For this review, take the finished solid that the model builds, in its own axes (mm). A direction names the side the tool comes from. Give positions to 0.01 mm unless a question says otherwise; leave off trailing zeros. Loops run counter-clockwise (first coordinate to the right, second up) from the corner with the lowest first, then second, coordinate; pieces in that order, holes last. Notation, with made-up numbers: (56, 17.25) - (65, 17.25) arc R12 cw to (65, 26.25) - close; hole circle Ø8 at (62, 79). An arc over 180 degrees is marked (long way). Use CSV: the item, a comma, the result in double quotes. Start each with the question number.
1. Wall thickness on line 1 (X direction, y = 0.5, z = -18); line 2 (X direction, y = -1, z = -23.5); line 3 (X direction, y = 3, z = -22.5): over which ranges is each line inside the solid? List them lowest first.
2. For faces 1 (the cylindrical face through (0.37, -0.06, -45.34)), 2 (the cylindrical face through (12.476, -0.632, 52.395)), list the 3-axis set-ups (+Z, -Z, +X, -X, +Y, -Y) from which the entire face can be reached by the end or side of a thin tool; tool diameter is ignored.
3. Take a section at B-B on z = 2.5. Give the boundary of the cut face in (x, y).
4. Take a section at C-C on x = -10.5. Give the boundary of the cut face in (y, z), plus the area to 3 significant figures.
5. Mouldability with a two-part tool opening along Y and no side actions: class faces 3 (the cylindrical face through (0.37, -0.06, 48.66)), 4 (the flat face through (32, -4, 25)), 5 (the cylindrical face through (-15.524, -0.632, 52.395)) as pulls with the +Y half, pulls with the -Y half, needs draft (parallel to the pull), parting line crosses it, or undercut.
6. Take a section at A-A on z = 23.5. Give the boundary of the cut face in (x, y), plus the area to 3 significant figures.
7. Take a section at D-D on x = 47. Give the boundary of the cut face in (y, z).
8. For pin 1 (4 mm diameter, centred on x = 0, z = -47, fed in from +Y); pin 2 (2 mm diameter, centred on x = -14, y = 0, fed in from +Z); pin 3 (3 mm diameter, centred on y = 0, z = -36.5, fed in from +X); pin 4 (1.5 mm diameter, centred on x = -40, y = 1, fed in from +Z), all flat-tipped, find the tip position at first contact; note any pin that passes through.
```python
from build123d import *

# Parameters (mm, degrees)
SKETCH_2_R                  = 40
EXTRUDE_1_DEPTH             = 4
HOLE_WIZARD_M3_1_D          = 3.4
HOLE_WIZARD_M4_1_AT_2_COUNT = 2
HOLE_WIZARD_M4_1_AT_2_PITCH = 28
HOLE_WIZARD_M4_3_D          = 3.3
HOLE_WIZARD_M4_3_DEPTH      = 15
HOLE_WIZARD_M4_3_TIP        = 0.991420021
HOLE_WIZARD_M4_2_D          = 4.3


with BuildPart() as part:
    # 草图2 → 凸台-拉伸1 (new, symmetric)
    with BuildSketch(Plane(origin=(0, 0, 0), x_dir=(1, 0, 0), z_dir=(0, 1, 0))):
        Polygon((23, 61.852813742), (-23, 61.852813742), (-74.618795027, 10.234018716), (-35, -60), (35, -60), (74.618795027, 10.234018716), align=None)
        with Locations(Location((0, 0, 0), (0, 0, 270))):
            Circle(SKETCH_2_R, mode=Mode.SUBTRACT)
    extrude(amount=EXTRUDE_1_DEPTH, both=True)

    # M3 间隙孔1 (through all)
    with Locations(Plane(origin=(0, 4, 0), x_dir=(1, 0, 0), z_dir=(0, 1, 0))):
        with Locations((0, 47), (40.703193978, 23.5), (40.703193978, -23.5), (0, -47), (-40.703193978, -23.5), (-40.703193978, 23.5)):
            Hole(HOLE_WIZARD_M3_1_D / 2)

    # 草图7 → Hole Wizard M4 _1 (revolve, cut)
    with BuildSketch(Plane(origin=(38.820162287, 0, -46.032651455), x_dir=(-0.7071067811865476, 0, -0.7071067811865476), z_dir=(0, 1, 0))):
        Polygon((0, 0), (0, 12.991420021), (1.65, 12), (1.65, 0), align=None)
    hole_wizard_m4_1 = revolve(axis=Axis((43.310290348, 0, -50.522779516), (-0.7071067811865476, 0, 0.7071067811865476)), mode=Mode.SUBTRACT)

    # Hole Wizard M4 _1 at 2: Hole Wizard M4 _1 ×2
    with Locations(*[Vector(0.7071067811865476, 0, 0.7071067811865476) * (i * HOLE_WIZARD_M4_1_AT_2_PITCH) for i in range(1, HOLE_WIZARD_M4_1_AT_2_COUNT)]):
        add(hole_wizard_m4_1, mode=Mode.SUBTRACT)

    # 镜向1: Hole Wizard M4 _1 across plane
    add(hole_wizard_m4_1.mirror(Plane(origin=(0, 0, 0), x_dir=(0, 0, 1), z_dir=(1, 0, 0))), mode=Mode.SUBTRACT)

    # 镜向1 copy 1 sketch → 镜向1 copy 1 (revolve, cut)
    with BuildSketch(Plane(origin=(-58.61915216, 0, -26.233661582), x_dir=(0.7071067811865476, 0, -0.7071067811865476), z_dir=(0, 1, 0))):
        Polygon((0, 0), (0, -12.991420021), (1.65, -12), (1.65, 0), align=None)
    revolve(axis=Axis((-63.109280221, 0, -30.723789643), (-0.7071067811865476, 0, -0.7071067811865476)), mode=Mode.SUBTRACT)

    # M4 螺纹孔3
    with Locations(Plane.XY.offset(60)):
        with Locations((14, 0), (-14, 0)):
            Hole(HOLE_WIZARD_M4_3_D / 2, depth=HOLE_WIZARD_M4_3_DEPTH)
            with Locations((0, 0, -(HOLE_WIZARD_M4_3_DEPTH + HOLE_WIZARD_M4_3_TIP / 2))):  # 118° drill point
                Cone(0, HOLE_WIZARD_M4_3_D / 2, HOLE_WIZARD_M4_3_TIP, mode=Mode.SUBTRACT)

    # M4 间隙孔2 (through all)
    with Locations(Plane(origin=(0, 4, 0), x_dir=(1, 0, 0), z_dir=(0, 1, 0))):
        with Locations((0, 56), (0, -56)):
            Hole(HOLE_WIZARD_M4_2_D / 2)


solid = part.part
```
Check result:
1,line 1,"x = -66.85 to -52.61, -49.27 to -35.72, 35.72 to 49.27, 52.61 to 66.85"
1,line 2,"x = -61.35 to -57.74, -54.03 to -42.4, -39 to -32.37, 32.37 to 39, 42.4 to 54.03, 57.74 to 61.35"
1,line 3,"x = -62.35 to -42.08, -39.33 to -33.07, 33.07 to 39.33, 42.08 to 62.35"
2,face 1,"+Y, -Y"
2,face 2,"+Z"
3,outline,"(-67.44, -4) - (-39.92, -4) - (-39.92, 4) - (-67.44, 4) - close; (39.92, -4) - (67.44, -4) - (67.44, 4) - (39.92, 4) - close"
4,outline,"(-4, -61.85) - (4, -61.85) - (4, -38.6) - (-4, -38.6) - close; (-4, 38.6) - (4, 38.6) - (4, 60) - (-4, 60) - close"
4,area,"357 mm²"
5,face 3,"needs draft"
5,face 4,"pulls with the -Y half"
5,face 5,"undercut"
6,outline,"(-55.59, -4) - (-42.4, -4) - (-42.4, 4) - (-55.59, 4) - close; (-39, -4) - (-32.37, -4) - (-32.37, 4) - (-39, 4) - close; (32.37, -4) - (39, -4) - (39, 4) - (32.37, 4) - close; (42.4, -4) - (55.59, -4) - (55.59, 4) - (42.4, 4) - close"
6,area,"317 mm²"
7,outline,"(-4, -37.85) - (4, -37.85) - (4, 38.73) - (-4, 38.73) - close"
8,pin 1,"stops at y = 4"
8,pin 2,"stops at z = 44.61"
8,pin 3,"stops at x = 49.85"
8,pin 4,"stops at z = 52.47"
